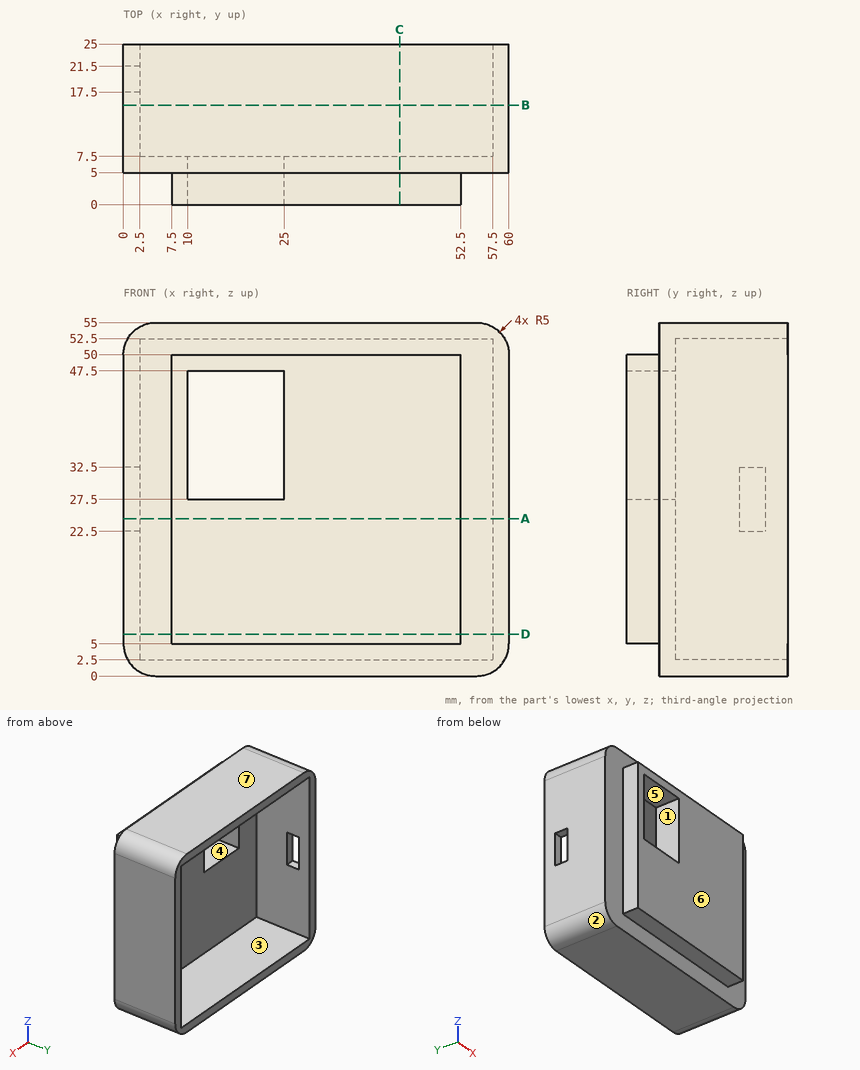
Answer from the drawing. Dimensions are ordinates in mm from the lowest x, y and z of the part. A direction names the side the tool comes from. Give positions to 0.01 mm unless a question says otherwise; leave off trailing zeros. Order: outer loops, then holes, each group sorted by start corner. A loop starts at its lowest first (then second) coordinate and runs counter-clockwise, first axis right, second up. Notation, with made-up numbers: (23, -28) - (76, -28) arc R7 cw to (76, -24) - close; hole circle Ø4 at (88, 11.5). An arc over 180 degrees is marked (long way). One line per item, written item: value. Start each with the question number.
1. For a pull along Z with two mould halves and no side action, classify the marked faces 4, 5, 6 and 7 as released by +Z, released by -Z, zero draft, split by the parting line, or undercut.
2. Consider line 1 (Z direction, x = 52, y = 10.25); line 2 (X direction, y = 3.5, z = 43); line 3 (X direction, y = 14.75, z = 41). Determine where each line is inside the solid, lowest interval first.
3. Section B-B, the plane y = 15.5 is taken. Write down the section's boundary in (x, z), then the cut area to 3 significant figures.
4. Section C-C, the plane x = 43 is taken. Write down the section's boundary in (y, z).
5. Which of the six approach directions +Z, -Z, +X, -X, +Y, -Y give full straight-line access (tool end or side, diameter ignored) to the marked faces 1, 2 and 3?
6. Section A-A, the plane z = 24.5 is taken. Write down the section's boundary in (x, y), then the cut area to 4 significant figures.
7. Each of these flat-tipped pins is pushed along its axis until it touches: pin 1 Ø2 at (x, y) = (16, 3) entering from -Z; pin 2 Ø2 at (x, z) = (1, 27.5) entering from -Y; pin 3 Ø1.2 at (x, y) = (1, 20) entering from -Z. Where does it stop, or does it pass through?
8. Section D-D, the plane z = 6.5 is taken. Write down the section's boundary in (x, y).
Filled sheet:
1. face 4: undercut
1. face 5: undercut
1. face 6: zero draft
1. face 7: released by +Z
2. line 1: 0 to 2.5, 52.5 to 55
2. line 2: 7.5 to 10, 25 to 52.5
2. line 3: 0 to 2.5, 57.5 to 60
3. outline: (0, 5) arc R5 ccw to (5, 0) - (55, 0) arc R5 ccw to (60, 5) - (60, 50) arc R5 ccw to (55, 55) - (5, 55) arc R5 ccw to (0, 50) - close; hole (2.5, 2.5) - (57.5, 2.5) - (57.5, 52.5) - (2.5, 52.5) - close
3. area: 529 mm²
4. outline: (0, 5) - (5, 5) - (5, 0) - (25, 0) - (25, 2.5) - (7.5, 2.5) - (7.5, 52.5) - (25, 52.5) - (25, 55) - (5, 55) - (5, 50) - (0, 50) - close
5. face 1: +Y, -Y
5. face 2: -Z, -X, +Y, -Y
5. face 3: +Y
6. outline: (0, 5) - (7.5, 5) - (7.5, 0) - (52.5, 0) - (52.5, 5) - (60, 5) - (60, 25) - (57.5, 25) - (57.5, 7.5) - (2.5, 7.5) - (2.5, 17.5) - (0, 17.5) - close; (0, 21.5) - (2.5, 21.5) - (2.5, 25) - (0, 25) - close
6. area: 452.5 mm²
7. pin 1: z = 5
7. pin 2: y = 5
7. pin 3: z = 1.33
8. outline: (0, 5) - (7.5, 5) - (7.5, 0) - (52.5, 0) - (52.5, 5) - (60, 5) - (60, 25) - (57.5, 25) - (57.5, 7.5) - (2.5, 7.5) - (2.5, 25) - (0, 25) - close
